Source: CAD feature listing. Evaluate the final solid. Frame: model axes, mm. A direction names the side the tool comes from. Round coordinates to 2 decimals unless told otherwise and drop trailing zeros. Order: outer loops, then holes, each group sorted by start corner. A loop starts at its lowest first (then second) coordinate and runs counter-clockwise, first axis right, second up. Notation, with made-up numbers: M -37,27.25 L -25,27.25 A17 cw -25,45.25 Z; hole C -28.5,-6.5 d1. An arc over 180 degrees is marked long. Use CSV: the item, a comma, the result in double quotes. Start each with the question number.
```python
from build123d import *

# Parameters (mm, degrees)
SKETCH2_W           = 11.43
SKETCH2_H           = 11.43
BOSS_EXTRUDE1_DEPTH = 5.08
BOSS_EXTRUDE2_DEPTH = 83.82
SKETCH4_W           = 7.62
SKETCH4_H           = 5.08
BOSS_EXTRUDE3_DEPTH = 7.62
SKETCH5_R           = 2.1717
CUT_EXTRUDE1_DEPTH  = 5.08
SKETCH6_R           = 2.1717
CUT_EXTRUDE2_DEPTH  = 5.08


with BuildPart() as part:
    # Sketch2 → Boss-Extrude1 (new body)
    with BuildSketch(Plane(origin=(0, 0, 0), x_dir=(1, 0, 0), z_dir=(0, 1, 0))):
        with Locations((4.433171137, -5.341620142)):
            Rectangle(SKETCH2_W, SKETCH2_H)
    extrude(amount=BOSS_EXTRUDE1_DEPTH)

    # Sketch3 → Boss-Extrude2 (add)
    with BuildSketch(Plane(origin=(0, 5.08, 0), x_dir=(1, 0, 0), z_dir=(0, 1, 0))):
        Polygon((-1.281828863, -11.056620142), (2.528171137, -11.056620142), (2.528171137, -3.436620142), (10.148171137, -3.436620142), (10.148171137, 0.373379858), (2.528171137, 0.373379858), (-1.281828863, 0.373379858), (-1.281828863, -3.436620142), align=None)
    extrude(amount=BOSS_EXTRUDE2_DEPTH)

    # Sketch4 → Boss-Extrude3 (add)
    with BuildSketch(Plane(origin=(2.528171137, 0, 0), x_dir=(0, 0, -1), z_dir=(1, 0, 0))):
        with Locations((-7.246620142, 86.36)):
            Rectangle(SKETCH4_W, SKETCH4_H)
    extrude(amount=BOSS_EXTRUDE3_DEPTH)

    # Sketch5 → Cut-Extrude1 (cut)
    with BuildSketch(Plane(origin=(0, 88.9, 0), x_dir=(1, 0, 0), z_dir=(0, 1, 0))):
        with Locations(Location((6.338171137, -7.246620142, 0), (0, 0, 270))):
            Circle(SKETCH5_R)
    extrude(amount=-CUT_EXTRUDE1_DEPTH, mode=Mode.SUBTRACT)

    # Sketch6 → Cut-Extrude2 (cut)
    with BuildSketch(Plane(origin=(0, 5.08, 0), x_dir=(1, 0, 0), z_dir=(0, 1, 0))):
        with Locations(Location((6.338171137, -7.246620142, 0), (0, 0, 270))):
            Circle(SKETCH6_R)
    extrude(amount=-CUT_EXTRUDE2_DEPTH, mode=Mode.SUBTRACT)


solid = part.part
```
(1) Section A-A on z = 7.25. Return loops of the section in (x, y).
(2) Reachability of faces 1 (the face through (-1.282, 44, 5)), 2 (the face through (4.6, 83.82, 5.6)) from +Z, -Z, +X, -X, +Y, -Y: full face, straight path, thin tool, end or side. Return the list, or none.
(3) Section C-C on y = 73. Return loops of the section in (x, z).
(4) Section B-B on x = 5. Return loops of the section in (y, z), plus the area to 3 significant figures.
(5) Contact query for a flat-ended pin moving along its axis: P1, Ø4, axis at y = 57.5, z = 6.5, coming from the +X side. Output: stop coordinate, or through.
(6) Line query: line 1 along Y through (x, z) = (3, 6.5); line 2 along X through (y, z) = (72, 8.75); line 3 along Z through (x, y) = (8.5, 72.5). Output: solid intervals per line, ascending.
(7) Draft query along Z for faces 3 (the face through (2.528, 44, 7)), 4 (the face through (6.434, 86.396, 5.077)), 5 (the face through (2, 34, 11.057)). Return one class per face: pulls with the +Z half, pulls with the -Z half, needs draft (parallel to the pull), parting line crosses it, or undercut.
Results below:
1,outline,"M -1.28,0 L 4.17,0 L 4.17,5.08 L 2.53,5.08 L 2.53,83.82 L 4.17,83.82 L 4.17,88.9 L -1.28,88.9 Z; M 8.51,0 L 10.15,0 L 10.15,5.08 L 8.51,5.08 Z; M 8.51,83.82 L 10.15,83.82 L 10.15,88.9 L 8.51,88.9 Z"
2,face 1,"+Z, -Z, -X, +Y, -Y"
2,face 2,"+Z, +X"
3,outline,"M -1.28,-0.37 L 10.15,-0.37 L 10.15,3.44 L 2.53,3.44 L 2.53,11.06 L -1.28,11.06 Z"
4,outline,"M 0,-0.37 L 88.9,-0.37 L 88.9,5.54 L 83.82,5.54 L 83.82,3.44 L 5.08,3.44 L 5.08,5.54 L 0,5.54 Z; M 0,8.96 L 5.08,8.96 L 5.08,11.06 L 0,11.06 Z; M 83.82,8.96 L 88.9,8.96 L 88.9,11.06 L 83.82,11.06 Z"
4,area,"381 mm2"
5,P1,"stops at x = 2.53"
6,line 1,"y = 0 to 5.08, 83.82 to 88.9"
6,line 2,"x = -1.28 to 2.53"
6,line 3,"z = -0.37 to 3.44"
7,face 3,"needs draft"
7,face 4,"undercut"
7,face 5,"pulls with the +Z half"
